Here's the drawing with two shaded views (mm, measured from the low corner). I have some questions. A direction names the side the tool comes from. Coordinates: 2 decimals unless noted, no trailing zeros. Order: outer loops, then holes, each group sorted by start corner. A loop starts at its lowest first (then second) coordinate and runs counter-clockwise, first axis right, second up. Notation, with made-up numbers: (-4.5, 78) -> (20.5, 78) arc R19 ccw to (20.5, 88) -> close; hole circle Ø1 at (44.25, 36). An arc over 180 degrees is marked (long way). Answer in a Markdown table with one row per item. Add a question column.
1. If I drill on line 1 along Z through (x, y) = (21, 3.5); line 2 along Y through (x, z) = (17.5, 4.5); line 3 along X through (y, z) = (5.25, 11.5) (1 decimal), over which ranges is the centre line in solid material (lowest first)? Write a range as [from, to].
2. Imagine slicing it at C-C on z = 2.25. Write out the boundary of the cut face in (x, y), plus the area to 3 significant figures.
3. We'd pull the mould along X, two halves only. Please class the marked faces 1 and 2: pulls with the +X half, pulls with the -X half, needs draft (parallel to the pull), parting line crosses it, or undercut.
4. Will these pins go through, and if not, where does the flat tip stop? pin 1 (4.5 mm diameter, centred on x = 31, y = 5.5, fed in from +Z); pin 2 (1.5 mm diameter, centred on x = 18.5, z = 2, fed in from +Y); pin 3 (2.5 mm diameter, centred on x = 22, z = 2.5, fed in from -Y); pin 4 (1.5 mm diameter, centred on x = 33, y = 8.5, fed in from -Z).
5. Imagine slicing it at A-A on z = 11. Write out the boundary of the cut face in (x, y).
6. On a 3-axis mill with a long thin cutter (end or side, diameter ignored), from which of +Z, -Z, +X, -X, +Y, -Y can I reach the whole of each face in a straight line? I mean the marked faces 3 and 4. Say none if no direction works.
7. Imagine slicing it at B-B on y = 4.25. Write out the boundary of the cut face in (x, z).
8. Imagine slicing it at D-D on x = 18. Write out the boundary of the cut face in (y, z).
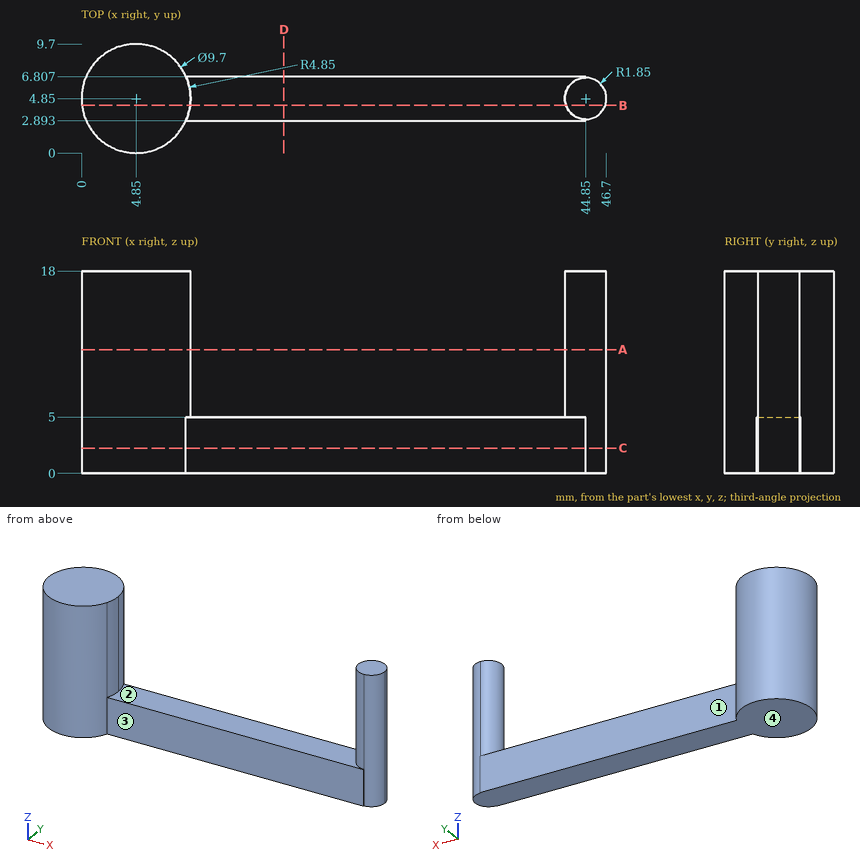
Answers follow:
| question | item | result |
|---|---|---|
| 1 | line 1 | z = [0, 5] |
| 1 | line 2 | y = [2.89, 6.81] |
| 1 | line 3 | x = [0, 9.7], [43, 46.7] |
| 2 | outline | (9.29, 2.89) -> (44.85, 2.89) -> (44.85, 3) arc R1.85 ccw to (44.85, 6.7) -> (44.85, 6.81) -> (9.29, 6.81) arc R4.85 ccw (long way) to start |
| 2 | area | 217 mm² |
| 3 | face 1 | needs draft |
| 3 | face 2 | undercut |
| 4 | pin 1 | stops at z = 5 |
| 4 | pin 2 | stops at y = 6.81 |
| 4 | pin 3 | stops at y = 2.89 |
| 4 | pin 4 | passes through |
| 5 | outline | circle Ø9.7 at (4.85, 4.85); circle Ø3.7 at (44.85, 4.85) |
| 6 | face 3 | +Z, -Z, +X, -Y |
| 6 | face 4 | -Z, +X, -X, +Y, -Y |
| 7 | outline | (0.04, 0) -> (46.6, 0) -> (46.6, 18) -> (43.1, 18) -> (43.1, 5) -> (9.66, 5) -> (9.66, 18) -> (0.04, 18) -> close |
| 8 | outline | (2.89, 0) -> (6.81, 0) -> (6.81, 5) -> (2.89, 5) -> close |
